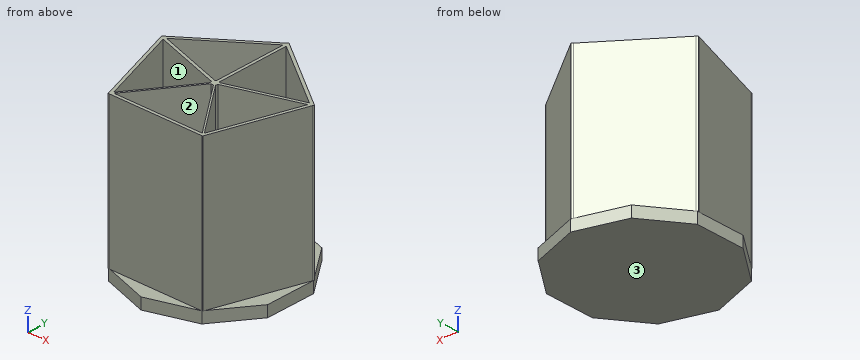
from build123d import *

# Parameters (mm, degrees)
F1_DEPTH = 101.6
F3_DEPTH = 7.62


with BuildPart() as f1:
    # F0 (on Top) → F1 (new body)
    with BuildSketch(Plane.XY):
        Polygon((1.007135, 2.090003), (1.007135, 51.900107), (-0.983909, 51.876503), (-1.0051, 2.090003), (0.00407, 2.820986), align=None)
        Polygon((52.457931, 17.016923), (51.435437, 17.760554), (49.010532, 16.973795), (49.67954, 15.127026), (52.098265, 15.911781), align=None)
        Polygon((-1.665072, 1.611959), (-49.016407, 17.019628), (-49.671557, 15.169454), (-2.321688, -0.237738), (-2.68166, 0.875603), align=None)
        Polygon((-49.016407, 17.019628), (-51.426483, 17.803844), (-52.441647, 17.067025), (-52.080348, 15.953252), (-49.671557, 15.169454), align=None)
        Polygon((49.67954, 15.127026), (49.010532, 16.973795), (1.663114, 1.611959), (2.684175, 0.867862), (2.323179, -0.237738), align=None)
        Polygon((1.663114, 1.611959), (1.007135, 2.090003), (0.00407, 2.820986), (-1.0051, 2.090003), (-1.665072, 1.611959), (-2.68166, 0.875603), (-2.321688, -0.237738), (-1.891828, -1.567235), (-1.661426, -2.279834), (-0.896572, -2.280937), (0.970708, -2.283631), (1.654842, -2.284618), (1.849318, -1.689005), (2.323179, -0.237738), (2.684175, 0.867862), align=None)
        Polygon((-0.983909, 51.876503), (-0.982828, 54.416503), (-51.426483, 17.803844), (-49.016407, 17.019628), align=None)
        Polygon((51.435437, 17.760554), (1.007135, 54.435669), (1.007135, 51.900107), (49.010532, 16.973795), align=None)
        Polygon((31.710784, -44.631538), (30.218665, -42.575976), (-30.193032, -42.554206), (-31.682195, -44.601329), align=None)
        Polygon((30.218665, -42.575976), (31.085375, -41.964973), (1.849318, -1.689005), (1.654842, -2.284618), (0.970708, -2.283631), align=None)
        Polygon((32.588472, -44.035659), (52.098265, 15.911781), (49.67954, 15.127026), (31.085375, -41.964973), align=None)
        Polygon((-49.671557, 15.169454), (-52.080348, 15.953252), (-32.667992, -43.889094), (-31.17694, -41.838673), align=None)
        Polygon((-1.891828, -1.567235), (-31.17694, -41.838673), (-30.193032, -42.554206), (-0.896572, -2.280937), (-1.661426, -2.279834), align=None)
        Polygon((1.007135, 54.435669), (0.026342, 55.148972), (-0.982828, 54.416503), (-0.983909, 51.876503), (1.007135, 51.900107), align=None)
        Polygon((-31.17694, -41.838673), (-32.667992, -43.889094), (-32.437065, -44.600969), (-31.682195, -44.601329), (-30.193032, -42.554206), align=None)
        Polygon((32.394438, -44.631864), (32.588472, -44.035659), (31.085375, -41.964973), (30.218665, -42.575976), (31.710784, -44.631538), align=None)
    extrude(amount=F1_DEPTH)

    # F2 (on Top) → F3 (join)
    with BuildSketch(Plane.XY):
        Polygon((-0.484477, -54.871911), (31.86095, -44.677077), (52.036577, -17.417118), (52.336, 16.495588), (32.64485, 44.10754), (0.484477, 54.871911), (-31.86095, 44.677077), (-52.036577, 17.417118), (-52.336, -16.495588), (-32.64485, -44.10754), align=None)
    extrude(amount=-F3_DEPTH)


solid = f1.part
Geometry: final body of the model. Coordinates: model frame, mm. Face numbers are marked on the shaded views. Give positions to 0.01 mm unless a question says otherwise; leave off trailing zeros. Write each loop counter-clockwise with the first axis right and the second up, starting at its lowest first coordinate (ties: lowest second). Pieces come first, ordered by that corner, then holes.
(1) Mould query, pull axis Y, two halves, no side actions, for the marked faces 1, 2 and 3. Classes: released by +Y, released by -Y, zero draft, split by the parting line, or undercut.
(2) First-contact query: P1, Ø14.5, axis at x = -24.5, y = 21, coming from the +Z side; P2, Ø4, axis at x = 24.5, z = 71, coming from the +Y side; P3, Ø1.5, axis at x = 26, z = 63.5, coming from the +Y side. Flat tips, straight axial feed; report the tip coordinate or a pass-through.
(3) Cut plane D-D, the plane y = -48. Return loops of the section in (x, z).
(4) Cut plane B-B, the plane z = 63.5. Give the number of separate pieces and of enclosed holes in the cut face, then the cut area to 3 significant figures.
(5) Cut plane C-C, the plane x = 42. Return loops of the section in (y, z).
(6) Cut plane A-A, the plane x = -5.5. Return loops of the section in (y, z).
(7) Ray query, line 1 (Y direction, x = -17.5, z = 10); line 2 (X direction, y = 36.5, z = 16.5); line 3 (Y direction, x = 24.5, z = 57). Return the intervals inside material, ascending.
Values follow:
1. face 1: undercut
1. face 2: undercut
1. face 3: zero draft
2. P1: stops at z = 0
2. P2: stops at y = 38.8
2. P3: stops at y = 36.8
3. outline: (-21.02, -7.62) - (21.32, -7.62) - (21.32, 0) - (-21.02, 0) - close
4. separate pieces: 1
4. enclosed holes: 5
4. area: 1,080 mm2
5. outline: (-30.98, -7.62) - (30.99, -7.62) - (30.99, 0) - (24.62, 0) - (24.62, 101.6) - (22.07, 101.6) - (22.07, 0) - (14.7, 0) - (14.7, 101.6) - (12.64, 101.6) - (12.64, 0) - (-8.45, 0) - (-8.45, 101.6) - (-15.12, 101.6) - (-15.12, 0) - (-30.98, 0) - close
6. outline: (-53.19, -7.62) - (52.99, -7.62) - (52.99, 0) - (51.14, 0) - (51.14, 101.6) - (48.6, 101.6) - (48.6, 0) - (2.86, 0) - (2.86, 101.6) - (0.8, 101.6) - (0.8, 0) - (-6.53, 0) - (-6.53, 101.6) - (-8.61, 101.6) - (-8.61, 0) - (-42.56, 0) - (-42.56, 101.6) - (-44.61, 101.6) - (-44.61, 0) - (-53.19, 0) - close
7. line 1: y = -44.61 to -42.56, -25.11 to -23.03, 4.7 to 6.76, 39.89 to 42.43
7. line 2: x = -25.67 to -22.17, -0.99 to 1.01, 22.17 to 25.67
7. line 3: y = -44.63 to -42.57, -34.7 to -32.89, 6.96 to 9.02, 34.81 to 37.35
